```python
from build123d import *

# Parameters (mm, degrees)
SKETCH1_R           = 16
BOSS_EXTRUDE1_DEPTH = 7


with BuildPart() as part:
    # Sketch1 → Boss-Extrude1 (new body)
    with BuildSketch(Plane(origin=(0, 0, 0), x_dir=(1, 0, 0), z_dir=(0, 1, 0))):
        with BuildLine():
            Line((2, -36), (2, -16.68052757))
            ThreePointArc((2, -16.68052757), (11.879393924, -11.879393924), (16.68052757, -2))
            Line((16.68052757, -2), (44, -2))
            Line((44, -2), (44, 2))
            Line((44, 2), (16.68052757, 2))
            ThreePointArc((16.68052757, 2), (-11.879393924, 11.879393924), (-2, -16.68052757))
            Line((-2, -16.68052757), (-2, -36))
            Line((-2, -36), (2, -36))
        make_face()
        with Locations(Location((0, 0, 0), (0, 0, 270))):
            Circle(SKETCH1_R, mode=Mode.SUBTRACT)
    extrude(amount=BOSS_EXTRUDE1_DEPTH)


solid = part.part
```
Read the model definition and answer for the solid it produces. Units are mm, in the model's axes. A direction names the side the tool comes from. Coordinates: 2 decimals unless noted, no trailing zeros. Order: outer loops, then holes, each group sorted by start corner. A loop starts at its lowest first (then second) coordinate and runs counter-clockwise, first axis right, second up. Notation, with made-up numbers: (58.25, 3) - (93.25, 3) arc R27 ccw to (93.25, 41) - close; hole circle Ø2 at (38, -30.5). An arc over 180 degrees is marked (long way). Answer as a JSON object with one key per item and string values. Group by question number.
Item 1: The mould has two halves that part along Z. Classify faces 6 (the face through (44, 3, 0)), 7 (the face through (11.77, 3.45, 11.99)), 8 (the face through (-15.62, 3.45, -3.47)): +Z half, -Z half, draft (parallel to the pull), parting line (faces both ways), or undercut.
Item 2: A tool of negligible diameter and unlimited length cuts with its end or side. For faces 1 (the face through (16, 0, 4)), 2 (the face through (-11.502, 3.451, -12.246)), 3 (the face through (-2, 3, 26)), 4 (the face through (31, 3, -2)), 5 (the face through (2, 3, 26)), from which of +Z, -Z, +X, -X, +Y, -Y can it reach the whole face along a straight path? Write none if from no direction.
Item 3: Flat-ended cylindrical pins translate along their axes: P1, Ø3.5, axis at y = 3.5, z = 31, coming from the -X side; P2, Ø1.5, axis at x = 9, y = 5, coming from the +Z side; P3, Ø12, axis at x = 19.5, z = 18.5, coming from the -Y side; P4, Ø2, axis at x = 36, y = 4, coming from the -Z side. Find the tip coordinate at first contact, or state that the pin passes through.
Item 4: Section C-C (y = 2) is taken. Give the vertices of the cut face in (x, z), plus the area to 3 significant figures.
Item 5: Section B-B (x = 0) is taken. Give the vertices of the cut face in (y, z).
Item 6: Consider probe 1 along X at (y, z) = (1.5, 0); probe 2 along Z at (x, y) = (0.5, 5.75); probe 3 along X at (y, z) = (2.5, 23.5). Determine where each line is inside the solid, lowest interval first. Write a range as from..to.
Item 7: Section A-A (z = 0) is taken. Give the vertices of the cut face in (x, y), plus the area to 3 significant figures.
Item 8: Section D-D (x = 37) is taken. Give the vertices of the cut face in (y, z), plus the area to 3 significant figures.
Results are:
{
 "1": {"face 6": "draft", "face 7": "+Z half", "face 8": "undercut"},
 "2": {"face 1": "+Z, -Z, +X, -X, -Y", "face 2": "+Y, -Y", "face 3": "+Z, -X, +Y, -Y", "face 4": "-Z, +X, +Y, -Y", "face 5": "+Z, +X, +Y, -Y"},
 "3": {"P1": "stops at x = -2", "P2": "stops at z = 14.63", "P3": "passes through", "P4": "stops at z = -2"},
 "4": {"outline": "(-2, 16.68) arc R16.8 ccw (long way) to (16.68, -2) - (44, -2) - (44, 2) - (16.68, 2) arc R16.8 ccw to (2, 16.68) - (2, 36) - (-2, 36) - close; hole circle Ø32 at (0, 0)", "area": "268 mm^2"},
 "5": {"outline": "(0, -16.8) - (7, -16.8) - (7, -16) - (0, -16) - close; (0, 16) - (7, 16) - (7, 36) - (0, 36) - close"},
 "6": {"probe 1": "x = -16.8..-16, 16..44", "probe 2": "z = -16.79..-15.99, 15.99..36", "probe 3": "x = -2..2"},
 "7": {"outline": "(-16.8, 0) - (-16, 0) - (-16, 7) - (-16.8, 7) - close; (16, 0) - (44, 0) - (44, 7) - (16, 7) - close", "area": "202 mm^2"},
 "8": {"outline": "(0, -2) - (7, -2) - (7, 2) - (0, 2) - close", "area": "28.0 mm^2"}
}
